Could you check a few things on this model? Use its own coordinates, in mm. Face numbers are marked on the shaded views. A direction names the side the tool comes from. Round coordinates to 2 decimals unless told otherwise and drop trailing zeros. Loops run counter-clockwise (first coordinate to the right, second up) from the corner with the lowest first, then second, coordinate; pieces in that order, holes last. Notation, with made-up numbers: (64.5, -26.5) -> (90.5, -26.5) arc R14 cw to (90.5, -0.5) -> close; hole circle Ø10 at (61, -19). An arc over 180 degrees is marked (long way). Use CSV: the item, a comma, the result in double quotes. Start each with the question number.
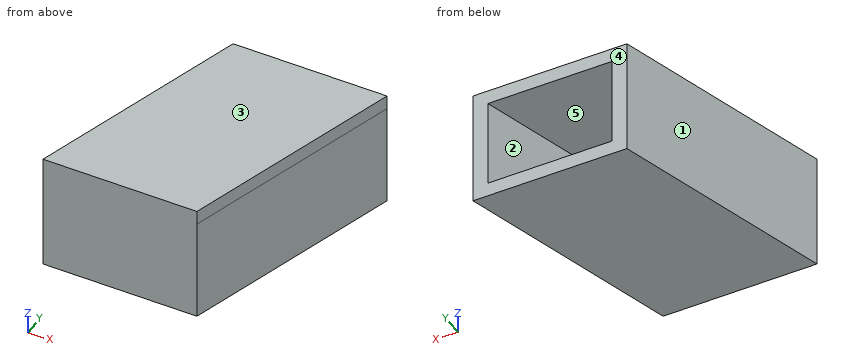
```python
from build123d import *

# Parameters (mm, degrees)
F1_DEPTH = 15.8
F3_DEPTH = 2.5
F4_START = -18.3
F4_DEPTH = 2.5


with BuildPart() as f1:
    # F0 (on Top) → F1 (new body)
    with BuildSketch(Plane.XY):
        Polygon((21.8094058029, 0), (0, 0), (11.0354576108, 35), (8.4141347979, 35), (-3.8825179684, -4), (23.1695334603, -4), (35.4661862265, 35), (32.8448634137, 35), align=None)
    extrude(amount=-F1_DEPTH)

    # F2 (on face) → F3 (join)
    with BuildSketch(Plane(origin=(0, 0, -15.8), x_dir=(1, 0, 0), z_dir=(0, 0, -1))):
        Polygon((11.0354576108, -35), (32.8448634137, -35), (21.8094058029, 0), (0, 0), align=None)
        Polygon((32.8448634137, -35), (35.4661862265, -35), (23.1695334603, 4), (-3.8825179684, 4), (8.4141347979, -35), (11.0354576108, -35), (0, 0), (21.8094058029, 0), align=None)
    extrude(amount=F3_DEPTH)

    # F3_face (on face) → F4 (join)
    with BuildSketch(Plane(origin=(15.7918341291, 15.5, -18.3), x_dir=(1, 0, 0), z_dir=(0, 0, -1)).offset(F4_START)):
        Polygon((19.6743520975, -19.5), (7.3776993312, 19.5), (-19.6743520975, 19.5), (-7.3776993312, -19.5), align=None)
    extrude(amount=-F4_DEPTH)


solid = f1.part
```
1. If I drill on L1, parallel to Z at x = 19.5, y = 21; L2, parallel to Y at x = 20, z = -15.5; L3, parallel to X at y = 29, z = -3.5, over which ranges is the centre line in solid material (lowest first)?
2. Will these pins go through, and if not, where does the flat tip stop? pin 1 (8 mm diameter, centred on y = 27.5, z = 0, fed in from +X); pin 2 (6 mm diameter, centred on y = 11, z = -15, fed in from -X); pin 3 (10 mm diameter, centred on y = 29, z = -2.5, fed in from -X).
3. For the marked faces 4 and 5, which set-ups out of +Z, -Z, +X, -X, +Y, -Y let a thin tool reach every point of the face, with its end or its side?
4. Suppose I cut it at A-A (z = -3.5). List the corners of the cut face in (x, y) for me.
5. We'd pull the mould along X, two halves only. Please class the marked faces 1, 2 and 3: pulls with the +X half, pulls with the -X half, needs draft (parallel to the pull), parting line crosses it, or undercut.
6. Suppose I cut it at B-B (x = 19). List the corners of the cut face in (y, z) for me.
7. Suppose I cut it at C-C (y = 26.5). List the corners of the cut face in (x, z) for me, then the cut area to 3 significant figures.
Geometry check:
1,L1,"z = -18.3 to -15.8, 0 to 2.5"
1,L2,"y = -4 to 0"
1,L3,"x = 6.52 to 9.14, 30.95 to 33.57"
2,pin 1,"stops at x = 34.36"
2,pin 2,"stops at x = -0.1"
2,pin 3,"stops at x = 4.95"
3,face 4,"+Z, -Z, +X, -X, +Y"
3,face 5,"none"
4,outline,"(-3.88, -4) -> (23.17, -4) -> (35.47, 35) -> (32.84, 35) -> (21.81, 0) -> (0, 0) -> (11.04, 35) -> (8.41, 35) -> close"
5,face 1,"pulls with the -X half"
5,face 2,"undercut"
5,face 3,"needs draft"
6,outline,"(-4, -18.3) -> (35, -18.3) -> (35, -15.8) -> (0, -15.8) -> (0, 0) -> (35, 0) -> (35, 2.5) -> (-4, 2.5) -> close"
7,outline,"(5.73, -18.3) -> (32.79, -18.3) -> (32.79, 2.5) -> (5.73, 2.5) -> close; hole (8.36, -15.8) -> (30.16, -15.8) -> (30.16, 0) -> (8.36, 0) -> close"
7,area,"218 mm²"
